from build123d import *

# Parameters (mm, degrees)
BOSS_EXTRU_1_DEPTH      = 5
ESQUISSE3_R             = 2.5
ENL_V_MAT_EXTRU_1_DEPTH = 5
ESQUISSE5_W             = 50
ESQUISSE5_H             = 8
ENL_V_MAT_EXTRU_3_DEPTH = 2.5


with BuildPart() as part:
    # Esquisse2 → Boss.-Extru.1 (new body)
    with BuildSketch(Plane.XY):
        Polygon((0, 0), (0, 8), (50, 8), (50, 13), (80, 13), (80, 0), align=None)
    extrude(amount=BOSS_EXTRU_1_DEPTH)

    # Esquisse3 → Enlèv. mat.-Extru.1 (cut)
    with BuildSketch(Plane.XY.offset(5)):
        with Locations((5, 4)):
            Circle(ESQUISSE3_R)
        with Locations((45, 4)):
            Circle(ESQUISSE3_R)
    extrude(amount=-ENL_V_MAT_EXTRU_1_DEPTH, mode=Mode.SUBTRACT)

    # Esquisse5 → Enlèv. mat.-Extru.3 (cut)
    with BuildSketch(Plane(origin=(0, 0, 0), x_dir=(-1, 0, 0), z_dir=(0, 0, -1))):
        with Locations((-25, 4)):
            Rectangle(ESQUISSE5_W, ESQUISSE5_H)
    extrude(amount=-ENL_V_MAT_EXTRU_3_DEPTH, mode=Mode.SUBTRACT)


solid = part.part
Could you check a few things on this model? Use its own coordinates, in mm. A direction names the side the tool comes from. Coordinates: 2 decimals unless noted, no trailing zeros. Write each loop counter-clockwise with the first axis right and the second up, starting at its lowest first coordinate (ties: lowest second). Pieces come first, ordered by that corner, then holes. Notation, with made-up numbers: (87.5, -39) - (100.5, -39) arc R20 cw to (100.5, -1) - close; hole circle Ø11 at (-24, 73.25). An arc over 180 degrees is marked (long way). Write item = value, one per line.
1) Suppose I cut it at C-C on z = 3.35. Please give me the cut outline in (x, y), plus the area to 3 significant figures.
Result set:
outline = (0, 0) - (80, 0) - (80, 13) - (50, 13) - (50, 8) - (0, 8) - close; hole circle Ø5 at (5, 4); hole circle Ø5 at (45, 4)
area = 751 mm2
2) Suppose I cut it at A-A on y = 4. Please give me the cut outline in (x, z), plus the area to 3 significant figures.
Result set:
outline = (0, 2.5) - (2.5, 2.5) - (2.5, 5) - (0, 5) - close; (7.5, 2.5) - (42.5, 2.5) - (42.5, 5) - (7.5, 5) - close; (47.5, 2.5) - (50, 2.5) - (50, 0) - (80, 0) - (80, 5) - (47.5, 5) - close
area = 250 mm2
3) For faces 1 (the flat face through (25, 4, 2.5)), 2 (the flat face through (0, 4, 4)), which set-ups out of +Z, -Z, +X, -X, +Y, -Y let a thin tool reach every point of the face, with its end or its side?
Result set:
face_1 = -Z, -X, +Y, -Y
face_2 = +Z, -Z, -X, +Y, -Y
4) We'd pull the mould along Y, two halves only. Please class faces 3 (the flat face through (80, 7, 2)), 4 (the cylindrical face through (7.385, 4.751, 3.768)), 5 (the flat face through (25, 8, 4)): +Y half, -Y half, draft (parallel to the pull), parting line (faces both ways), or undercut.
Result set:
face_3 = draft
face_4 = undercut
face_5 = +Y half
5) Suppose I cut it at D-D on x = 17. Please give me the cut outline in (y, z), plus the area to 3 significant figures.
Result set:
outline = (0, 2.5) - (8, 2.5) - (8, 5) - (0, 5) - close
area = 20.0 mm2
6) Will these pins go through, and if not, where does the flat tip stop? pin 1 Ø2.5 at (x, y) = (12.5, 2.5) entering from -Z; pin 2 Ø3 at (x, z) = (31.5, 3.5) entering from +Y; pin 3 Ø2 at (y, z) = (5.5, 1) entering from -X; pin 4 Ø4 at (x, y) = (5, 4) entering from -Z.
Result set:
pin_1 = 2.5
pin_2 = 8
pin_3 = 50
pin_4 = through
7) Suppose I cut it at B-B on x = 45. Please give me the cut outline in (y, z), plus the area to 3 significant figures.
Result set:
outline = (0, 2.5) - (1.5, 2.5) - (1.5, 5) - (0, 5) - close; (6.5, 2.5) - (8, 2.5) - (8, 5) - (6.5, 5) - close
area = 7.50 mm2
8) Please list where these lines run through material, in increasing order: line 1 (Y direction, x = 5, z = 3.35); line 2 (Y direction, x = 27, z = 4.2); line 3 (Z direction, x = 15.5, y = 1.25). Write a range as [from, to].
Result set:
line_1 = [0, 1.5], [6.5, 8]
line_2 = [0, 8]
line_3 = [2.5, 5]
